from build123d import *

# Parameters (mm, degrees)
SKETCH1_W           = 8
SKETCH1_H           = 8
SKETCH1_R           = 3
BOSS_EXTRUDE2_DEPTH = 22
CUT_EXTRUDE1_REACH  = 25.749
SKETCH2_R           = 1.5


with BuildPart() as part:
    # Sketch1 → Boss-Extrude2 (new body)
    with BuildSketch(Plane(origin=(0, 0, 0), x_dir=(1, 0, 0), z_dir=(0, 1, 0))):
        Rectangle(SKETCH1_W, SKETCH1_H)
        with Locations(Location((0, 0, 0), (0, 0, 270))):
            Circle(SKETCH1_R, mode=Mode.SUBTRACT)
    extrude(amount=BOSS_EXTRUDE2_DEPTH)

    # Cut-Extrude1: up to this face of the body (flat: up to its plane)
    cut_extrude1_end = Plane(part.part.faces().sort_by_distance((-4, 11, 0))[0])
    # Sketch2 → Cut-Extrude1 (cut, up to the picked face)
    with BuildSketch(Plane(origin=(4, 0, 0), x_dir=(0, 0, -1), z_dir=(1, 0, 0)), mode=Mode.PRIVATE) as cut_extrude1_sk1:
        with Locations((0, 18)):
            Circle(SKETCH2_R)
    cut_extrude1_tool1 = split(extrude(cut_extrude1_sk1.sketch, amount=-CUT_EXTRUDE1_REACH, mode=Mode.PRIVATE), bisect_by=cut_extrude1_end, keep=Keep.BOTH, mode=Mode.PRIVATE)
    # Sketch2 → Cut-Extrude1 (cut, up to the picked face)
    with BuildSketch(Plane(origin=(4, 0, 0), x_dir=(0, 0, -1), z_dir=(1, 0, 0)), mode=Mode.PRIVATE) as cut_extrude1_sk2:
        with Locations((0, 4)):
            Circle(SKETCH2_R)
    cut_extrude1_tool2 = split(extrude(cut_extrude1_sk2.sketch, amount=-CUT_EXTRUDE1_REACH, mode=Mode.PRIVATE), bisect_by=cut_extrude1_end, keep=Keep.BOTH, mode=Mode.PRIVATE)
    add(cut_extrude1_tool1.solids().sort_by(Axis((4, 18, 0), (-1, 0, 0)))[0], mode=Mode.SUBTRACT)
    add(cut_extrude1_tool2.solids().sort_by(Axis((4, 4, 0), (-1, 0, 0)))[0], mode=Mode.SUBTRACT)


solid = part.part
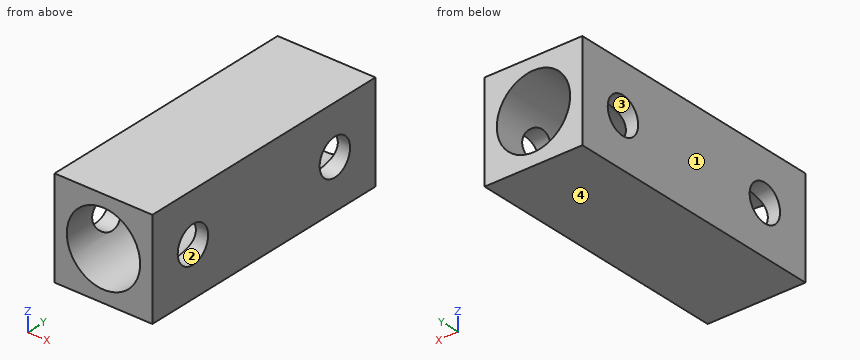
For this review, take the finished solid that the model builds, in its own axes (mm). Face numbers are marked on the shaded views. Give positions to 0.01 mm unless a question says otherwise; leave off trailing zeros. Loops run counter-clockwise (first coordinate to the right, second up) from the corner with the lowest first, then second, coordinate; pieces in that order, holes last. Notation, with made-up numbers: M -28.5,74 L 3.5,74 A12 ccw 3.5,83 Z; hole C 70,-13 d7. An arc over 180 degrees is marked long. Put each result on its own line as item: value. Start each with the question number.
(1) Add section C-C, the plane z = 1. Write out the cut boundary in (x, y).
(2) Add section B-B, the plane y = 4. Write out the cut boundary in (x, z).
(3) Add section D-D, the plane y = 13.75. Write out the cut boundary in (x, z).
(4) The part is to be moulded in two halves that separate along Z. For the marked faces 1, 2, 3 and 4, say which applies: +Z half, -Z half, draft (parallel to the pull), parting line (faces both ways), or undercut.
(5) For pin 1 (2.5 mm diameter, centred on y = 4, z = 0, fed in from +X), flat-tipped, find the tip position at first contact; note if it passes through.
(6) Wall thickness on L1, parallel to Y at x = 3.65, z = 0; L2, parallel to X at y = 15, z = 0; L3, parallel to Z at x = -3.2, y = 4: over which ranges is each line inside the solid? List them lowest first.
(7) Add section A-A, the plane x = 0. Write out the cut boundary in (y, z), then the cut area to 3 significant figures.
Result:
1. outline: M -4,0 L -2.83,0 L -2.83,2.88 L -4,2.88 Z; M -4,5.12 L -2.83,5.12 L -2.83,16.88 L -4,16.88 Z; M -4,19.12 L -2.83,19.12 L -2.83,22 L -4,22 Z; M 2.83,0 L 4,0 L 4,2.88 L 2.83,2.88 Z; M 2.83,5.12 L 4,5.12 L 4,16.88 L 2.83,16.88 Z; M 2.83,19.12 L 4,19.12 L 4,22 L 2.83,22 Z
2. outline: M -4,-4 L 4,-4 L 4,-1.5 L 2.6,-1.5 A3 cw -2.6,-1.5 L -4,-1.5 Z; M -4,1.5 L -2.6,1.5 A3 cw 2.6,1.5 L 4,1.5 L 4,4 L -4,4 Z
3. outline: M -4,-4 L 4,-4 L 4,4 L -4,4 Z; hole C 0,0 d6
4. face 1: draft
4. face 2: undercut
4. face 3: undercut
4. face 4: -Z half
5. pin 1: passes through
6. L1: y = 0 to 2.5, 5.5 to 16.5, 19.5 to 22
6. L2: x = -4 to -3, 3 to 4
6. L3: z = -4 to -1.5, 1.5 to 4
7. outline: M 0,-4 L 22,-4 L 22,-3 L 0,-3 Z; M 0,3 L 22,3 L 22,4 L 0,4 Z
7. area: 44.0 mm^2
